from build123d import *
from OCP.BRepFilletAPI import BRepFilletAPI_MakeChamfer

# Parameters (mm, degrees)
BOSS_EXTRUDE1_DEPTH      = 1
BOSS_EXTRUDE1_DEPTH_BACK = 1
SKETCH3_R                = 12
SKETCH3_R_2              = 6
CHAMFER1_SIZE            = 0.254
CHAMFER1_SIZE2           = 0.439940905
CHAMFER2_SIZE            = 0.536952942


with BuildPart() as part:
    # Sketch3 → Boss-Extrude1 (new, two sides: drawn at the far end of the back side and taken through both)
    with BuildSketch(Plane.XY.offset(-BOSS_EXTRUDE1_DEPTH_BACK)):
        Circle(SKETCH3_R)
        Circle(SKETCH3_R_2, mode=Mode.SUBTRACT)
    extrude(amount=BOSS_EXTRUDE1_DEPTH + BOSS_EXTRUDE1_DEPTH_BACK)

    # Chamfer1: one chamfer whose edges measure the first distance from different faces: ONE call of the kernel's chamfer builder (chamfer() names one face for all edges)
    chamfer1_edges_1 = [part.edges().sort_by_distance(p)[0] for p in [
        (-12, 0, 1),
    ]]
    chamfer1_side_1 = [part.faces().sort_by_distance(p)[0] for p in [
        (-12, 0, 0.5),
    ]]
    chamfer1_edges_2 = [part.edges().sort_by_distance(p)[0] for p in [
        (-12, 0, -1),
    ]]
    chamfer1_side_2 = [part.faces().sort_by_distance(p)[0] for p in [
        (-12, 0, -0.5),
    ]]
    chamfer1 = BRepFilletAPI_MakeChamfer(part.part.solid().wrapped)
    for e in chamfer1_edges_1:
        chamfer1.Add(CHAMFER1_SIZE, CHAMFER1_SIZE2, e.wrapped, chamfer1_side_1[0].wrapped)  # the first distance lies on this face
    for e in chamfer1_edges_2:
        chamfer1.Add(CHAMFER1_SIZE, CHAMFER1_SIZE2, e.wrapped, chamfer1_side_2[0].wrapped)  # the first distance lies on this face
    add(Compound.cast(chamfer1.Shape()), mode=Mode.REPLACE)

    # Sketch4 → Cut-Revolve1 (revolve, cut)
    with BuildSketch(Plane(origin=(0, 0, 0), x_dir=(0, 0, -1), z_dir=(1, 0, 0)), mode=Mode.PRIVATE) as cut_revolve1_sk:
        with BuildLine():
            Line((-1, 5.9492), (-1, 6.0508))
            ThreePointArc((-1, 6.0508), (0, 6), (1, 6.0508))
            Line((1, 6.0508), (1, 5.9492))
            Line((1, 5.9492), (-1, 5.9492))
        make_face()
    revolve(cut_revolve1_sk.sketch.rotate(Axis((0, 0, 1), (0, 0, -1)), 90), axis=Axis((0, 0, 1), (0, 0, -1)), mode=Mode.SUBTRACT)

    # Chamfer2
    # the kernel refuses this chamfer: 0.536952942, 0.254 mm, written as the material it takes off along each edge
    with BuildSketch(Plane(origin=(0, 0, -1), x_dir=(1, 0, 0), z_dir=(0, 1, 0))) as chamfer2_piece_1:
        with BuildLine():
            Line((6.0508 + CHAMFER2_SIZE, 0), (6.028453739, -0.251168371))
            ThreePointArc((6.028453739, -0.251168371), (6.038361074, -0.130738), (6.0508, 0))
            Line((6.0508, 0), (6.0508 + CHAMFER2_SIZE, 0))
        make_face()
    revolve(axis=Axis((0, 0, -1), (0, 0, -1)), mode=Mode.SUBTRACT)
    with BuildSketch(Plane(origin=(0, 0, 1), x_dir=(1, 0, 0), z_dir=(0, 1, 0))) as chamfer2_piece_2:
        with BuildLine():
            Line((6.0508 + CHAMFER2_SIZE, 0), (6.028453739, 0.251168371))
            ThreePointArc((6.028453739, 0.251168371), (6.038361074, 0.130738), (6.0508, 0))
            Line((6.0508, 0), (6.0508 + CHAMFER2_SIZE, 0))
        make_face()
    revolve(axis=Axis((0, 0, 1), (0, 0, -1)), mode=Mode.SUBTRACT)


solid = part.part
The listing builds one solid part. Answer for the finished solid, in the listing's coordinates (mm). Coordinates: 2 decimals unless noted, no trailing zeros. Write each loop counter-clockwise with the first axis right and the second up, starting at its lowest first coordinate (ties: lowest second). Pieces come first, ordered by that corner, then holes. Notation, with made-up numbers: M 67.5,77 L 119.5,77 A9 cw 119.5,93 Z; hole C 21,-18 d1. An arc over 180 degrees is marked long. Write each question's results on one line, items separated by ' | '.
Item 1: The part is cut by section C-C on z = -0.05. Determine the outline of the cut face in (x, y).
Answer below:
outline: C 0,0 d24; hole C 0,0 d12
Item 2: Given P1, Ø1, axis at y = -7.5, z = 0, coming from the +X side, flat-ended and moving along its own axis, determine where the tip first touches the part or whether it passes through.
Answer below:
P1: x = 9.75
Item 3: The part is cut by section A-A on y = 0. Determine the outline of the cut face in (x, z).
Answer below:
outline: M -12,-0.75 L -11.56,-1 L -6.59,-1 L -6.03,-0.75 A9.87 ccw -6.03,0.75 L -6.59,1 L -11.56,1 L -12,0.75 Z; M 6.03,-0.75 L 6.59,-1 L 11.56,-1 L 12,-0.75 L 12,0.75 L 11.56,1 L 6.59,1 L 6.03,0.75 A9.87 ccw Z
Item 4: Consider probe 1 along X at (y, z) = (5, 0.55); probe 2 along Y at (x, z) = (-4, 0.6); probe 3 along X at (y, z) = (-1, 0). Determine where each line is inside the solid, lowest interval first. Write a range as [from, to].
Answer below:
probe 1: [-10.91, -3.34], [3.34, 10.91] | probe 2: [-11.31, -4.5], [4.5, 11.31] | probe 3: [-11.96, -5.92], [5.92, 11.96]
